Source: CAD feature listing. Evaluate the final solid. Frame: model axes, mm. A direction names the side the tool comes from. Round coordinates to 2 decimals unless told otherwise and drop trailing zeros. Order: outer loops, then holes, each group sorted by start corner. A loop starts at its lowest first (then second) coordinate and runs counter-clockwise, first axis right, second up. Notation, with made-up numbers: (0, 55.5) -> (47, 55.5) arc R16 cw to (47, 65.5) -> close; hole circle Ø11 at (66.5, 7.25). An arc over 180 degrees is marked (long way). One line per item, written item: value. Start each with the question number.
1) Section B-B (x = 154). Return the cut outline in (y, z).
2) Pin query (flat end, axial travel): P1, Ø1.6, axis at y = 100.5, z = 54.5, coming from the +X side; P2, Ø6, axis at x = 131, y = 85, coming from the -Z side. Return the tip coordinate at first contact, or that it passes through.
3) Section A-A (y = 35). Return the cut outline in (x, z).
4) Ray query, L1, parallel to X at y = 70, z = 47.5; L2, parallel to Y at x = 44, z = 24; L3, parallel to X at y = 89.5, z = 30.5. Return the intervals inside material, ascending.
5) Reachability of faces 1 (the face through (132, 76.2, 44)), 2 (the face through (13, 0, 44)) from +Z, -Z, +X, -X, +Y, -Y: full face, straight path, thin tool, end or side. Return the list, or none.
```python
from build123d import *

# Parameters (mm, degrees)
BOSS_EXTRUDE2_DEPTH = 88.9
CUT_EXTRUDE3_DEPTH  = 89.9
FILLET2_R           = 6.35
FILLET4_R           = 0.762


with BuildPart() as part:
    # Sketch1 → Boss-Extrude2 (new body)
    with BuildSketch(Plane.XY):
        Polygon((0, 0), (0, 101.6), (233.68, 101.6), (233.68, 76.2), (25.4, 76.2), (25.4, 0), align=None)
    extrude(amount=BOSS_EXTRUDE2_DEPTH)

    # Sketch8 → Cut-Extrude3 (cut, through all)
    with BuildSketch(Plane.XY.offset(88.9)):
        Polygon((228.6, 76.2), (228.6, 78.740000094), (230.178469436, 79.314515955), (230.178469436, 80.449652208), (231.371879071, 80.88401777), (232.101530561, 80.014452928), (233.68, 80.58896879), (233.68, 76.2), align=None)
        Polygon((228.6, 101.6), (233.68, 101.6), (233.68, 97.21103121), (232.101530561, 97.785547072), (231.371879071, 96.91598223), (230.178469436, 97.350347792), (230.178469436, 98.485484045), (228.6, 99.059999906), align=None)
        Polygon((228.6, 86.36), (228.6, 91.44), (230.178469436, 92.014515861), (230.178469436, 93.149652114), (231.371879071, 93.584017676), (232.101530561, 92.714452834), (233.68, 93.288968696), (233.68, 84.511031304), (232.101530561, 85.085547166), (231.371879071, 84.215982324), (230.178469436, 84.650347886), (230.178469436, 85.785484139), align=None)
    extrude(amount=-CUT_EXTRUDE3_DEPTH, mode=Mode.SUBTRACT)

    # Fillet2
    fillet2_edges = [part.edges().sort_by_distance(p)[0] for p in [
        (0, 101.6, 44.45),
        (25.4, 76.2, 44.45),
    ]]
    fillet(fillet2_edges, radius=FILLET2_R)

    # Fillet4
    fillet4_edges = [part.edges().sort_by_distance(p)[0] for p in [
        (228.6, 78.740000094, 44.45),
        (228.6, 99.059999906, 44.45),
        (228.6, 91.44, 44.45),
        (228.6, 86.36, 44.45),
    ]]
    fillet(fillet4_edges, radius=FILLET4_R)


solid = part.part
```
Findings:
1. outline: (76.2, 0) -> (101.6, 0) -> (101.6, 88.9) -> (76.2, 88.9) -> close
2. P1: x = 228.6
2. P2: z = 0
3. outline: (0, 0) -> (25.4, 0) -> (25.4, 88.9) -> (0, 88.9) -> close
4. L1: 0 to 25.4
4. L2: 76.2 to 101.6
4. L3: 0 to 228.6
5. face 1: +Z, -Z, +X, -Y
5. face 2: +Z, -Z, +X, -X, -Y
